The listing builds one solid part. Answer for the finished solid, in the listing's coordinates (mm). A direction names the side the tool comes from. Round coordinates to 2 decimals unless told otherwise and drop trailing zeros. Order: outer loops, then holes, each group sorted by start corner. A loop starts at its lowest first (then second) coordinate and runs counter-clockwise, first axis right, second up. Notation, with made-up numbers: (-3, 11.5) - (25, 11.5) arc R34 cw to (25, 47.5) - close; hole circle Ø11 at (-1.5, 15). An arc over 180 degrees is marked (long way). Use CSV: the item, a comma, the result in double quotes. Start each with the question number.
Item 1: Find section A-A, the plane x = 48. Give the vertices of the cut face in (y, z), plus the area to 3 significant figures.
Item 2: Find section C-C, the plane x = 66.5. Give the vertices of the cut face in (y, z), plus the area to 3 significant figures.
Item 3: For faces 1 (the cylindrical face through (10.61, 22.49, 3.04)), 2 (the cylindrical face through (13.04, 29.93, 3.04)), 3 (the flat face through (78, 27, 3)), 4 (the flat face through (6, 21, 3)), 5 (the flat face through (36, 2, 3)), determine the directions among +Z, -Z, +X, -X, +Y, -Y from which every point of the face is accessible in a straight line to the end or side of a thin tool.
Item 4: Determine the mould class of faces 6 (the flat face through (40, 17, 6)), 7 (the flat face through (13, 23.509, 3)), 8 (the flat face through (72.215, 4.437, 2.958)) for opening direction X: +X half, -X half, draft (parallel to the pull), parting line (faces both ways), or undercut.
Item 5: Find section B-B, the plane z = 2.1. Count the separate pieces of the cut face and the enclosed holes in it, plus the area to 3 significant figures.
Item 6: Straight lines are drawn through the part: line 1 along X through (y, z) = (9.5, 3.05); line 2 along Y through (x, z) = (45, 1.75); line 3 along X through (y, z) = (3, 5.35). For each, find the intervals that lie inside material, in ascending order. Write a range as [from, to].
Item 7: Find section D-D, the plane y = 11. Give the vertices of the cut face in (x, z).
Item 8: Flat-ended cylindrical pins translate along their axes: P1, Ø1, axis at y = 7.5, z = 2, coming from the +X side; P2, Ø3, axis at y = 2, z = 3.5, coming from the +X side; P3, Ø1.5, axis at y = 22.5, z = 3, coming from the -X side. Find the tip coordinate at first contact, or state that the pin passes through.
```python
from build123d import *

# Parameters (mm, degrees)
ESQUISSE1_W             = 82
ESQUISSE1_H             = 33
BOSS_EXTRU_1_DEPTH      = 6
ENL_V_MAT_EXTRU_1_DEPTH = 10
ESQUISSE3_W             = 6
ESQUISSE3_H             = 7
ENL_V_MAT_EXTRU_2_DEPTH = 89.594582227
CHANFREIN1_SIZE         = 13
CHANFREIN1_SIZE2        = 27.878589967
CHANFREIN2_SIZE         = 9
CHANFREIN2_SIZE2        = 19.300562285
ESQUISSE4_W             = 12
ESQUISSE4_H             = 3.2
ENL_V_MAT_EXTRU_3_DEPTH = 10
ESQUISSE5_R             = 3.070048726
ENL_V_MAT_EXTRU_4_DEPTH = 10
ESQUISSE6_W             = 6
ESQUISSE6_H             = 9
ENL_V_MAT_EXTRU_5_DEPTH = 89.594582227


with BuildPart() as part:
    # Esquisse1 → Boss.-Extru.1 (new body)
    with BuildSketch(Plane.XY):
        with Locations((41, 16.5)):
            Rectangle(ESQUISSE1_W, ESQUISSE1_H)
    extrude(amount=BOSS_EXTRU_1_DEPTH)

    # Esquisse2 → Enlèv. mat.-Extru.1 (cut)
    with BuildSketch(Plane.XY.offset(6)):
        Polygon((82, 33), (79, 33), (79, 27), (76, 27), (76, 19), (82, 19), align=None)
    extrude(amount=-ENL_V_MAT_EXTRU_1_DEPTH, mode=Mode.SUBTRACT)

    # Esquisse3 → Enlèv. mat.-Extru.2 (cut, through all)
    with BuildSketch(Plane.XY.offset(6)):
        with Locations((3, 21.5)):
            Rectangle(ESQUISSE3_W, ESQUISSE3_H)
    extrude(amount=-ENL_V_MAT_EXTRU_2_DEPTH, mode=Mode.SUBTRACT)

    # Chanfrein1
    chanfrein1_edges = [part.edges().sort_by_distance(p)[0] for p in [
        (0, 0, 3),
    ]]
    chanfrein1_side = [part.faces().sort_by_distance(p)[0] for p in [
        (0, 9, 3),
    ]]
    chamfer(chanfrein1_edges, length=CHANFREIN1_SIZE, length2=CHANFREIN1_SIZE2, reference=chanfrein1_side[0])

    # Chanfrein2
    chanfrein2_edges = [part.edges().sort_by_distance(p)[0] for p in [
        (82, 0, 3),
    ]]
    chanfrein2_side = [part.faces().sort_by_distance(p)[0] for p in [
        (82, 9.5, 3),
    ]]
    chamfer(chanfrein2_edges, length=CHANFREIN2_SIZE, length2=CHANFREIN2_SIZE2, reference=chanfrein2_side[0])

    # Esquisse4 → Enlèv. mat.-Extru.3 (cut)
    with BuildSketch(Plane.XY.offset(6)):
        with Locations((45, 8.4)):
            Rectangle(ESQUISSE4_W, ESQUISSE4_H)
        with Locations((67, 8.4)):
            Rectangle(ESQUISSE4_W, ESQUISSE4_H)
    extrude(amount=-ENL_V_MAT_EXTRU_3_DEPTH, mode=Mode.SUBTRACT)

    # Esquisse5 → Enlèv. mat.-Extru.4 (cut)
    with BuildSketch(Plane.XY.offset(6)):
        with Locations((13.110300044, 33)):
            Circle(ESQUISSE5_R)
        with BuildLine():
            Line((448.809841118, 61.994892284), (448.809841118, 59.994892284))
            ThreePointArc((448.809841118, 59.994892284), (447.809841118, 58.994892284), (446.809841118, 59.994892284))
            Line((446.809841118, 59.994892284), (446.809841118, 61.994892284))
            ThreePointArc((446.809841118, 61.994892284), (447.809841118, 62.994892284), (448.809841118, 61.994892284))
        make_face()
        with BuildLine():
            Line((442.809841118, 61.994892284), (442.809841118, 59.994892284))
            ThreePointArc((442.809841118, 59.994892284), (441.809841118, 58.994892284), (440.809841118, 59.994892284))
            Line((440.809841118, 59.994892284), (440.809841118, 61.994892284))
            ThreePointArc((440.809841118, 61.994892284), (441.809841118, 62.994892284), (442.809841118, 61.994892284))
        make_face()
        with BuildLine():
            Line((442.809841118, 86.994892284), (442.809841118, 84.994892284))
            ThreePointArc((442.809841118, 84.994892284), (441.809841118, 83.994892284), (440.809841118, 84.994892284))
            Line((440.809841118, 84.994892284), (440.809841118, 86.994892284))
            ThreePointArc((440.809841118, 86.994892284), (441.809841118, 87.994892284), (442.809841118, 86.994892284))
        make_face()
        with BuildLine():
            Line((442.809841118, 111.994892284), (442.809841118, 109.994892284))
            ThreePointArc((442.809841118, 109.994892284), (441.809841118, 108.994892284), (440.809841118, 109.994892284))
            Line((440.809841118, 109.994892284), (440.809841118, 111.994892284))
            ThreePointArc((440.809841118, 111.994892284), (441.809841118, 112.994892284), (442.809841118, 111.994892284))
        make_face()
        with BuildLine():
            Line((442.809841118, 136.994892284), (442.809841118, 134.994892284))
            ThreePointArc((442.809841118, 134.994892284), (441.809841118, 133.994892284), (440.809841118, 134.994892284))
            Line((440.809841118, 134.994892284), (440.809841118, 136.994892284))
            ThreePointArc((440.809841118, 136.994892284), (441.809841118, 137.994892284), (442.809841118, 136.994892284))
        make_face()
        with BuildLine():
            Line((448.809841118, 86.994892284), (448.809841118, 84.994892284))
            ThreePointArc((448.809841118, 84.994892284), (447.809841118, 83.994892284), (446.809841118, 84.994892284))
            Line((446.809841118, 84.994892284), (446.809841118, 86.994892284))
            ThreePointArc((446.809841118, 86.994892284), (447.809841118, 87.994892284), (448.809841118, 86.994892284))
        make_face()
        with BuildLine():
            Line((448.809841118, 111.994892284), (448.809841118, 109.994892284))
            ThreePointArc((448.809841118, 109.994892284), (447.809841118, 108.994892284), (446.809841118, 109.994892284))
            Line((446.809841118, 109.994892284), (446.809841118, 111.994892284))
            ThreePointArc((446.809841118, 111.994892284), (447.809841118, 112.994892284), (448.809841118, 111.994892284))
        make_face()
        with BuildLine():
            Line((448.809841118, 136.994892284), (448.809841118, 134.994892284))
            ThreePointArc((448.809841118, 134.994892284), (447.809841118, 133.994892284), (446.809841118, 134.994892284))
            Line((446.809841118, 134.994892284), (446.809841118, 136.994892284))
            ThreePointArc((446.809841118, 136.994892284), (447.809841118, 137.994892284), (448.809841118, 136.994892284))
        make_face()
        with BuildLine():
            Line((11.610300044, 23.509087354), (14.610300044, 23.509087354))
            ThreePointArc((14.610300044, 23.509087354), (15.610300044, 22.509087354), (14.610300044, 21.509087354))
            Line((14.610300044, 21.509087354), (11.610300044, 21.509087354))
            ThreePointArc((11.610300044, 21.509087354), (10.610300044, 22.509087354), (11.610300044, 23.509087354))
        make_face()
    extrude(amount=-ENL_V_MAT_EXTRU_4_DEPTH, mode=Mode.SUBTRACT)

    # Esquisse6 → Enlèv. mat.-Extru.5 (cut, through all)
    with BuildSketch(Plane.XY.offset(6)):
        with Locations((33, -0.5)):
            Rectangle(ESQUISSE6_W, ESQUISSE6_H)
    extrude(amount=-ENL_V_MAT_EXTRU_5_DEPTH, mode=Mode.SUBTRACT)


solid = part.part
```
Worked out:
1,outline,"(0, 0) - (6.8, 0) - (6.8, 6) - (0, 6) - close; (10, 0) - (33, 0) - (33, 6) - (10, 6) - close"
1,area,"179 mm²"
2,outline,"(1.77, 0) - (6.8, 0) - (6.8, 6) - (1.77, 6) - close; (10, 0) - (33, 0) - (33, 6) - (10, 6) - close"
2,area,"168 mm²"
3,face 1,"+Z, -Z"
3,face 2,"+Z, -Z, +Y"
3,face 3,"+Z, -Z, +X"
3,face 4,"+Z, -Z, -X"
3,face 5,"+Z, -Z, -Y"
4,face 6,"draft"
4,face 7,"undercut"
4,face 8,"+X half"
5,separate pieces,"1"
5,enclosed holes,"3"
5,area,"2,210 mm²"
6,line 1,"x = [7.51, 39], [51, 61], [73, 82]"
6,line 2,"y = [0, 6.8], [10, 33]"
6,line 3,"x = [21.45, 30], [36, 69.13]"
7,outline,"(4.29, 0) - (82, 0) - (82, 6) - (4.29, 6) - close"
8,P1,"stops at x = 79.86"
8,P2,"stops at x = 70.21"
8,P3,"stops at x = 6"
